from build123d import *

# Parameters (mm, degrees)
BOSS_EXTRUDE1_DEPTH     = 2
CUT_EXTRUDE2_DEPTH      = 2
WALL_MOUNT_HOLES_R      = 3
CUT_EXTRUDE3_DEPTH      = 2
STANDOFF_MOUNTS_R       = 2.6
BOSS_EXTRUDE3_DEPTH     = 4
ODROID_C1_MOUNT_HOLES_R = 1.7
CUT_EXTRUDE4_DEPTH      = 6


with BuildPart() as part:
    # Base plate → Boss-Extrude1 (new body)
    with BuildSketch(Plane(origin=(0, 0, 0), x_dir=(1, 0, 0), z_dir=(0, 1, 0))):
        Polygon((-13.872098625, 23.726545041), (71.127901375, 23.726545041), (71.10965601, -32.373454959), (-13.872098625, -32.373454959), align=None)
    extrude(amount=BOSS_EXTRUDE1_DEPTH)

    # Base Plate Hole → Cut-Extrude2 (cut)
    with BuildSketch(Plane(origin=(0, 0, 0), x_dir=(1, 0, 0), z_dir=(0, 1, 0))):
        Polygon((6.127901375, 3.726545041), (51.121395731, 3.726545041), (51.116159539, -12.373454959), (6.127901375, -12.373454959), align=None)
    extrude(amount=CUT_EXTRUDE2_DEPTH, mode=Mode.SUBTRACT)

    # Wall Mount Holes → Cut-Extrude3 (cut)
    with BuildSketch(Plane(origin=(0, 0, 0), x_dir=(1, 0, 0), z_dir=(0, 1, 0))):
        with Locations(Location((-3.872098625, 13.726545041, 0), (0, 0, 270))):
            Circle(WALL_MOUNT_HOLES_R)
        with Locations(Location((-3.872098625, -22.373454959, 0), (0, 0, 270))):
            Circle(WALL_MOUNT_HOLES_R)
        with Locations(Location((61.124648553, 13.726545041, 0), (0, 0, 270))):
            Circle(WALL_MOUNT_HOLES_R)
        with Locations(Location((61.112907774, -22.373454959, 0), (0, 0, 270))):
            Circle(WALL_MOUNT_HOLES_R)
    extrude(amount=CUT_EXTRUDE3_DEPTH, mode=Mode.SUBTRACT)

    # Standoff Mounts → Boss-Extrude3 (add)
    with BuildSketch(Plane(origin=(0, 2, 0), x_dir=(1, 0, 0), z_dir=(0, 1, 0))):
        with Locations(Location((-10.44034399, 20.276545041, 0), (0, 0, 270))):
            Circle(STANDOFF_MOUNTS_R)
        with Locations(Location((47.65965601, 20.276545041, 0), (0, 0, 270))):
            Circle(STANDOFF_MOUNTS_R)
        with Locations(Location((-10.44034399, -28.923454959, 0), (0, 0, 270))):
            Circle(STANDOFF_MOUNTS_R)
        with Locations(Location((47.65965601, -28.923454959, 0), (0, 0, 270))):
            Circle(STANDOFF_MOUNTS_R)
    extrude(amount=BOSS_EXTRUDE3_DEPTH)

    # Odroid C1 Mount Holes → Cut-Extrude4 (cut)
    with BuildSketch(Plane(origin=(0, 6, 0), x_dir=(1, 0, 0), z_dir=(0, 1, 0))):
        with Locations(Location((-10.44034399, -28.923454959, 0), (0, 0, 270))):
            Circle(ODROID_C1_MOUNT_HOLES_R)
        with Locations(Location((-10.44034399, 20.276545041, 0), (0, 0, 270))):
            Circle(ODROID_C1_MOUNT_HOLES_R)
        with Locations(Location((47.65965601, 20.276545041, 0), (0, 0, 270))):
            Circle(ODROID_C1_MOUNT_HOLES_R)
        with Locations(Location((47.65965601, -28.923454959, 0), (0, 0, 270))):
            Circle(ODROID_C1_MOUNT_HOLES_R)
    extrude(amount=-CUT_EXTRUDE4_DEPTH, mode=Mode.SUBTRACT)


solid = part.part
For this review, take the finished solid that the model builds, in its own axes (mm). A direction names the side the tool comes from. Give positions to 0.01 mm unless a question says otherwise; leave off trailing zeros. Loops run counter-clockwise (first coordinate to the right, second up) from the corner with the lowest first, then second, coordinate; pieces in that order, holes last. Notation, with made-up numbers: M 25.25,-28 L 69.25,-28 A12 ccw 69.25,-23 Z; hole C 19,48 d5. An arc over 180 degrees is marked long. Put each result on its own line as item: value. Start each with the question number.
(1) Add section B-B, the plane z = 22. Write out the cut boundary in (x, y), then the cut area to 3 significant figures.
(2) Wall thickness on L1, parallel to Z at x = 38, y = 0.7; L2, parallel to X at y = 0.7, z = 11; L3, parallel to Y at x = 7, z = 17: over which ranges is each line inside the solid? List them lowest first.
(3) Add section A-A, the plane y = 4.25. Write out the cut boundary in (x, z).
(4) The part is to be moulded in two halves that separate along X. For faces 4 (the flat face through (28, 1, -23.727)), 5 (the cylindrical face through (46.664, 3.972, 31.325)), 6 (the flat face through (-13.872, 1, 5)), say which applies: +X half, -X half, draft (parallel to the pull), parting line (faces both ways), or undercut.
(5) Add section C-C, the plane x = 41.5. Write out the cut boundary in (y, z), then the cut area to 3 significant figures.
(6) For pin 1 (8 mm diameter, centred on x = 61.11, z = 22.37, fed in from +Y); pin 2 (2 mm diameter, centred on y = 1, z = 6.5, fed in from +X); pin 3 (3.5 mm diameter, centred on x = -3.87, z = 22.37, fed in from +Y), all flat-tipped, find the tip position at first contact; note any pin that passes through.
(7) Machinability: for faces 1 (the flat face through (29, 2, 16)), 2 (the flat face through (47, 6, 31)), 3 (the flat face through (29, 1, 12.373)), which of the approach directions +Z, -Z, +X, -X, +Y, -Y give a long, thin tool a straight path to every point of the face, cutting with its end or side? Answer none if there is none.
(8) Add section D-D, the plane z = -1. Write out the cut boundary in (x, y).
Result:
1. outline: M -13.87,0 L -6.85,0 L -6.85,2 L -13.87,2 Z; M -0.9,0 L 58.14,0 L 58.14,2 L -0.9,2 Z; M 64.09,0 L 71.11,0 L 71.11,2 L 64.09,2 Z
1. area: 146 mm^2
2. L1: z = -23.73 to -3.73, 12.37 to 32.37
2. L2: x = -13.87 to 6.13, 51.12 to 71.12
2. L3: y = 0 to 2
3. outline: C -10.44,-20.28 d5.2; C -10.44,28.92 d5.2; C 47.66,-20.28 d5.2; C 47.66,28.92 d5.2; hole C -10.44,-20.28 d3.4; hole C -10.44,28.92 d3.4; hole C 47.66,-20.28 d3.4; hole C 47.66,28.92 d3.4
4. face 4: draft
4. face 5: undercut
4. face 6: -X half
5. outline: M 0,-23.73 L 2,-23.73 L 2,-3.73 L 0,-3.73 Z; M 0,12.37 L 2,12.37 L 2,32.37 L 0,32.37 Z
5. area: 80.0 mm^2
6. pin 1: stops at y = 2
6. pin 2: stops at x = 71.12
6. pin 3: passes through
7. face 1: +Y
7. face 2: +Z, -Z, +X, -X, +Y
7. face 3: +Y, -Y
8. outline: M -13.87,0 L 6.13,0 L 6.13,2 L -13.87,2 Z; M 51.12,0 L 71.12,0 L 71.12,2 L 51.12,2 Z
